Can you work these out from the model? Positions are in its coordinate system, mm. A direction names the side the tool comes from. Round coordinates to 2 decimals unless told otherwise and drop trailing zeros. Write each loop counter-clockwise with the first axis right and the second up, starting at its lowest first coordinate (ties: lowest second). Pieces come first, ordered by that corner, then holes. Notation, with made-up numbers: (39.25, 22.5) -> (97.25, 22.5) arc R9 cw to (97.25, 37.5) -> close; hole circle Ø6 at (-21, 8.5). An arc over 180 degrees is marked (long way). Write item = value, one per line. Start each with the question number.
1) Imagine slicing it at C-C, the plane y = -2. Please give me the cut outline in (x, z), then the cut area to 3 significant figures.
2) Imagine slicing it at D-D, the plane x = 9.5. Please give me the cut outline in (y, z).
3) If I drill on line 1 (Y direction, x = 15, z = 2.8); line 2 (X direction, y = -2, z = 3.5); line 3 (X direction, y = 1.5, z = 2.2), over which ranges is the centre line in solid material (lowest first)?
4) Thinking about a two-plate mould opening in Y: for faces 3 (the face through (0, 4, 3)), 4 (the face through (0, 0, 5.08)), 5 (the face through (0, 10.073, 3)), which applies, +Y half, -Y half, draft (parallel to the pull), parting line (faces both ways), or undercut?
5) Imagine slicing it at A-A, the plane z = 1.15. Please give me the cut outline in (x, y).
6) Imagine slicing it at B-B, the plane x = -8.5. Please give me the cut outline in (y, z), then the cut area to 3 significant figures.
7) For faces 1 (the face through (-9, -6.907, 3)), 2 (the face through (0, -10.073, 3)), which set-ups out of +Z, -Z, +X, -X, +Y, -Y let a thin tool reach every point of the face, with its end or its side?
from build123d import *

# Parameters (mm, degrees)
F1_DEPTH = 5.08


with BuildPart() as f1:
    # F0 (on Top) → F1 (new body)
    with BuildSketch(Plane.XY):
        Polygon((21.0098195821, 10.0732017308), (0, 10.0732017308), (-21.0098195821, 10.0732017308), (-21.0098195821, 0), (-21.0098195821, -10.0732017308), (0, -10.0732017308), (21.0098195821, -10.0732017308), (21.0098195821, 0), align=None)
        with BuildLine():
            Line((15.2537059039, -6.9073382765), (2.8924141151, -6.9073382765))
            ThreePointArc((2.8924141151, -6.9073382765), (1.4751092249, -7.3417596157), (0, -7.4884832563))
            ThreePointArc((0, -7.4884832563), (-1.4751092249, -7.3417596157), (-2.8924141151, -6.9073382765))
            Line((-2.8924141151, -6.9073382765), (-15.2537059039, -6.9073382765))
            Line((-15.2537059039, -6.9073382765), (-15.2537059039, -0.5080337272))
            Line((-15.2537059039, -0.5080337272), (-15.2537059039, 0))
            Line((-15.2537059039, 0), (-15.2537059039, 6.9073382765))
            Line((-15.2537059039, 6.9073382765), (-2.8924141151, 6.9073382765))
            ThreePointArc((-2.8924141151, 6.9073382765), (-1.4751092249, 7.3417596157), (0, 7.4884832563))
            ThreePointArc((0, 7.4884832563), (1.4751092249, 7.3417596157), (2.8924141151, 6.9073382765))
            Line((2.8924141151, 6.9073382765), (15.2537059039, 6.9073382765))
            Line((15.2537059039, 6.9073382765), (15.2537059039, 0.3525706587))
            Line((15.2537059039, 0.3525706587), (15.2537059039, 0))
            Line((15.2537059039, 0), (15.2537059039, -6.9073382765))
        make_face(mode=Mode.SUBTRACT)
        with BuildLine():
            ThreePointArc((-7.4884832563, 0), (-6.234467746, 4.1483482742), (-2.8924141151, 6.9073382765))
            Line((-2.8924141151, 6.9073382765), (-15.2537059039, 6.9073382765))
            Line((-15.2537059039, 6.9073382765), (-15.2537059039, 0))
            Line((-15.2537059039, 0), (-15.2537059039, -0.5080337272))
            Line((-15.2537059039, -0.5080337272), (-7.471230368, -0.5080337272))
            ThreePointArc((-7.471230368, -0.5080337272), (-7.4841687913, -0.2541632989), (-7.4884832563, 0))
        make_face()
        with BuildLine():
            ThreePointArc((7.4801788354, 0.3525706587), (7.4864068632, 0.176334223), (7.4884832563, 0))
            ThreePointArc((7.4884832563, 0), (6.234467746, -4.1483482742), (2.8924141151, -6.9073382765))
            Line((2.8924141151, -6.9073382765), (15.2537059039, -6.9073382765))
            Line((15.2537059039, -6.9073382765), (15.2537059039, 0))
            Line((15.2537059039, 0), (15.2537059039, 0.3525706587))
            Line((15.2537059039, 0.3525706587), (7.4801788354, 0.3525706587))
        make_face()
        with BuildLine():
            ThreePointArc((-2.8924141151, -6.9073382765), (-1.4751092249, -7.3417596157), (0, -7.4884832563))
            Line((0, -7.4884832563), (0, -0.5792839078))
            ThreePointArc((0, -0.5792839078), (-0.4096155795, -0.4096155795), (-0.5792839078, 0))
            Line((-0.5792839078, 0), (-7.4884832563, 0))
            ThreePointArc((-7.4884832563, 0), (-7.4841687913, -0.2541632989), (-7.471230368, -0.5080337272))
            ThreePointArc((-7.471230368, -0.5080337272), (-6.0900785235, -4.35755953), (-2.8924141151, -6.9073382765))
        make_face()
        with BuildLine():
            Line((0.5792839078, 0), (7.4884832563, 0))
            ThreePointArc((7.4884832563, 0), (7.4864068632, 0.176334223), (7.4801788354, 0.3525706587))
            ThreePointArc((7.4801788354, 0.3525706587), (6.1350562964, 4.2940034605), (2.8924141151, 6.9073382765))
            ThreePointArc((2.8924141151, 6.9073382765), (1.4751092249, 7.3417596157), (0, 7.4884832563))
            Line((0, 7.4884832563), (0, 0.5792839078))
            ThreePointArc((0, 0.5792839078), (0.4096155795, 0.4096155795), (0.5792839078, 0))
        make_face()
        with BuildLine():
            Line((-0.5792839078, 0), (0, 0))
            Line((0, 0), (0, 0.5792839078))
            ThreePointArc((0, 0.5792839078), (-0.4096155795, 0.4096155795), (-0.5792839078, 0))
        make_face()
        with BuildLine():
            Line((0, 0), (0.5792839078, 0))
            ThreePointArc((0.5792839078, 0), (0.4096155795, 0.4096155795), (0, 0.5792839078))
            Line((0, 0.5792839078), (0, 0))
        make_face()
        with BuildLine():
            ThreePointArc((0, -0.5792839078), (0.4096155795, -0.4096155795), (0.5792839078, 0))
            Line((0.5792839078, 0), (0, 0))
            Line((0, 0), (0, -0.5792839078))
        make_face()
        with BuildLine():
            Line((0, -0.5792839078), (0, 0))
            Line((0, 0), (-0.5792839078, 0))
            ThreePointArc((-0.5792839078, 0), (-0.4096155795, -0.4096155795), (0, -0.5792839078))
        make_face()
    extrude(amount=F1_DEPTH)


solid = f1.part
Reported:
q1.outline = (-21.01, 0) -> (-15.25, 0) -> (-15.25, 5.08) -> (-21.01, 5.08) -> close; (-7.22, 0) -> (0, 0) -> (0, 5.08) -> (-7.22, 5.08) -> close; (7.22, 0) -> (21.01, 0) -> (21.01, 5.08) -> (7.22, 5.08) -> close
q1.area = 136 mm²
q2.outline = (-10.07, 0) -> (0.35, 0) -> (0.35, 5.08) -> (-10.07, 5.08) -> close; (6.91, 0) -> (10.07, 0) -> (10.07, 5.08) -> (6.91, 5.08) -> close
q3.line_1 = -10.07 to 0.35, 6.91 to 10.07
q3.line_2 = -21.01 to -15.25, -7.22 to 0, 7.22 to 21.01
q3.line_3 = -21.01 to -7.34, 0 to 7.34, 15.25 to 21.01
q4.face_3 = undercut
q4.face_4 = draft
q4.face_5 = +Y half
q5.outline = (-21.01, -10.07) -> (21.01, -10.07) -> (21.01, 10.07) -> (-21.01, 10.07) -> close; hole (-15.25, -6.91) -> (-2.89, -6.91) arc R7.49 cw to (-7.47, -0.51) -> (-15.25, -0.51) -> close; hole (-7.49, 0) -> (-0.58, 0) arc R0.58 cw to (0, 0.58) -> (0, 7.49) arc R7.49 ccw to start; hole (0, -7.49) arc R7.49 ccw to (7.49, 0) -> (0.58, 0) arc R0.58 cw to (0, -0.58) -> close; hole (2.89, 6.91) arc R7.49 cw to (7.48, 0.35) -> (15.25, 0.35) -> (15.25, 6.91) -> close
q6.outline = (-10.07, 0) -> (-6.91, 0) -> (-6.91, 5.08) -> (-10.07, 5.08) -> close; (-0.51, 0) -> (10.07, 0) -> (10.07, 5.08) -> (-0.51, 5.08) -> close
q6.area = 69.8 mm²
q7.face_1 = +Z, -Z
q7.face_2 = +Z, -Z, +X, -X, -Y
